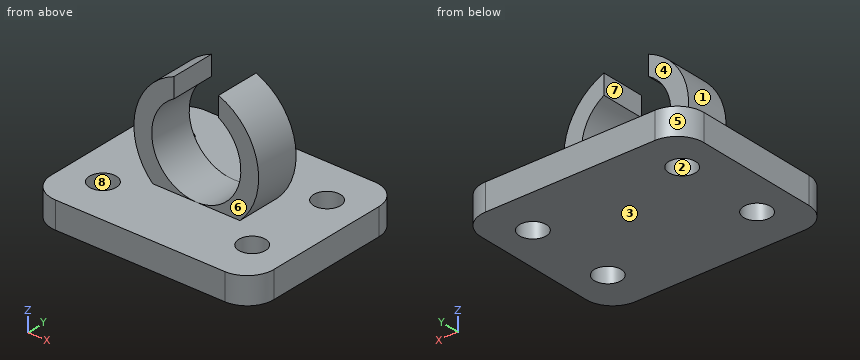
Autodesk Inventor part; units mm, degrees
ref_plane "YZ Plane" through (0, 0, 0) normal (1, 0, 0) x (0, 1, 0)
ref_plane "XZ Plane" through (0, 0, 0) normal (0, 1, 0) x (-1, 0, 0)
ref_plane "XY Plane" through (0, 0, 0) normal (0, 0, 1) x (1, 0, 0)
sketch "Szkic1" plane through (0, 0, 0) normal (0, 0, 1) x (1, 0, 0)
  line L0 (-12.5, -10) -> (12.5, -10)
  line L1 (12.5, -10) -> (12.5, 10)
  line L2 (12.5, 10) -> (-12.5, 10)
  line L3 (-12.5, 10) -> (-12.5, -10)
  line L4 (-12.5, -10) -> (12.5, 10) construction
  line L5 (12.5, -10) -> (-12.5, 10) construction
  point P0 (0, 0)
  dimension "d0" = 25
  dimension "d1" = 20
extrude "Wyciągnięcie proste1" add sketch "Szkic1" along normal blind 3
sketch "Szkic2" plane through (0, 0, 0) normal (0, 1, 0) x (-1, 0, 0)
  circle A0 centre (0, 8) radius 7
  line L0 (12.5, 3) -> (-12.5, 3)
  line L1 (12.5, 0) -> (-12.5, 0)
  circle A1 centre (0, 8) radius 5
  line L2 (4.899, 3) -> (-4.899, 3)
  point P0 (0, 0)
  point P1 (0, 0)
  dimension "d4" = 14
  dimension "d5" = 10
extrude "Wyciągnięcie proste2" add sketch "Szkic2" along normal mid plane 5 contours A0 L0 picked at (6.263, 8.5684)
sketch "Szkic3" plane through (-12.5, 10, 0) normal (0, 1, 0) x (1, 0, 0)
  line L0 (10, -16) -> (15, -16)
  line L1 (15, -16) -> (15, -12)
  line L2 (15, -12) -> (10, -12)
  line L3 (10, -12) -> (10, -16)
  line L4 (10, -16) -> (15, -12) construction
  line L5 (15, -16) -> (10, -12) construction
  circle A0 centre (12.5, -8) radius 5
  line L6 (25, 0) -> (0, 0)
  point P0 (12.5, 0)
  point P1 (12.5, -14)
  point P2 (12.5, -14)
  point P3 (12.5, 0)
  dimension "d8" = 5
  dimension "d9" = 4
  dimension "d10" = 6
extrude "Wyciągnięcie proste3" cut sketch "Szkic3" against normal blind 20 contours L3 A0 L1 L0 | L3 L2 L1 A0 picked at (12.3258, -12.3242)
sketch "Szkic5" plane through (0, 0, 0) normal (0, 0, -1) x (-1, 0, 0)
  line L0 (12.5, 10) -> (12.5, -10)
  line L1 (-12.5, 10) -> (12.5, 10)
  line L2 (-12.5, -10) -> (-12.5, 10)
  line L3 (-12.5, 0) -> (12.5, 0) construction
  line L4 (0, 10) -> (0, -10) construction
  line L5 (12.5, -10) -> (-12.5, -10)
  point P0 (0, 0)
  point P1 (8.375, 5)
  point P2 (8.375, -5)
  point P3 (-8.375, 5)
  point P4 (-8.375, -5)
  dimension "d22" = 4.125
  dimension "d23" = 5
hole "Otwór2" at (-8.375, 5, 0) at (-8.375, -5, 0) at (8.375, 5, 0) at (8.375, -5, 0) direction (0, 0, 1) diameter 3 end through all
fillet "Zaokrąglenie1" radius 3 4 edges at (-12.5, -10, 1.5) (-12.5, 10, 1.5) (12.5, 10, 1.5) (12.5, -10, 1.5)
properties part number "uchwyt_przewody"
Could you check a few things on this model? Use its own coordinates, in mm. Face numbers are marked on the shaded views. A direction names the side the tool comes from. Round coordinates to 2 decimals unless told otherwise and drop trailing zeros. Loops run counter-clockwise (first coordinate to the right, second up) from the corner with the lowest first, then second, coordinate; pieces in that order, holes last. Notation, with made-up numbers: (23, -7.75) - (53, -7.75) arc R34 ccw to (53, 26.25) - close; hole circle Ø11 at (-36, -12.5). An arc over 180 degrees is marked (long way). Answer in a Markdown table with one row per item. Add a question column.
(1) If we section it at B-B (z = 8): Please give me the cut outline in (x, y).
(2) If we mould it in two halves opening along Z, with no side actions, what happens to the marked faces 1, 2 and 3? For each: pulls with the +Z half, pulls with the -Z half, needs draft (parallel to the pull), parting line crosses it, or undercut.
(3) I need wall thicknesses on line 1 along X through (y, z) = (-5, 1.35) (3 decimals); line 2 along Y through (x, z) = (-9.75, 2); line 3 along Z through (x, y) = (0.75, 3). Which ranges of each line are inside material? Lowest first, please.
(4) If we section it at C-C (z = 2.25): Please give me the cut outline in (x, y) (3 decimals).
(5) I'm going to push flat-ended pins straight in: pin 1 (2.5 mm diameter, centred on x = 8.375, y = 5, fed in from -Z); pin 2 (8 mm diameter, centred on x = 9, y = 2, fed in from -Z); pin 3 (1 mm diameter, centred on y = 2.5, z = 12.5, fed in from +X); pin 4 (3.5 mm diameter, centred on x = 3, z = 11, fed in from +Y). Where does each tip first touch, or does it pass through?
(6) If we section it at A-A (y = 5): Please give me the cut outline in (x, z) (3 decimals), plus the area to 3 significant figures.
(7) For the marked faces 4, 5, 6, 7 and 8, which set-ups out of +Z, -Z, +X, -X, +Y, -Y let a thin tool reach every point of the face, with its end or its side?
Model answer:
| question | item | result |
|---|---|---|
| 1 | outline | (-7, -2.5) - (-5, -2.5) - (-5, 2.5) - (-7, 2.5) - close; (5, -2.5) - (7, -2.5) - (7, 2.5) - (5, 2.5) - close |
| 2 | face 1 | undercut |
| 2 | face 2 | needs draft |
| 2 | face 3 | pulls with the -Z half |
| 3 | line 1 | x = -12.5 to -9.875, -6.875 to 6.875, 9.875 to 12.5 |
| 3 | line 2 | y = -9.99 to -5.6, -4.4 to 4.4, 5.6 to 9.99 |
| 3 | line 3 | z = 0 to 3 |
| 4 | outline | (-12.5, -7) arc R3 ccw to (-9.5, -10) - (9.5, -10) arc R3 ccw to (12.5, -7) - (12.5, 7) arc R3 ccw to (9.5, 10) - (-9.5, 10) arc R3 ccw to (-12.5, 7) - close; hole circle Ø3 at (-8.375, -5); hole circle Ø3 at (-8.375, 5); hole circle Ø3 at (8.375, -5); hole circle Ø3 at (8.375, 5) |
| 5 | pin 1 | passes through |
| 5 | pin 2 | stops at z = 0 |
| 5 | pin 3 | stops at x = 5.74 |
| 5 | pin 4 | stops at y = 2.5 |
| 6 | outline | (-12.5, 0) - (-9.875, 0) - (-9.875, 3) - (-12.5, 3) - close; (-6.875, 0) - (6.875, 0) - (6.875, 3) - (-6.875, 3) - close; (9.875, 0) - (12.5, 0) - (12.5, 3) - (9.875, 3) - close |
| 6 | area | 57.0 mm² |
| 7 | face 4 | +Z, +X, -X, +Y |
| 7 | face 5 | +Z, -Z, -X, +Y |
| 7 | face 6 | +Z, +X, -X, -Y |
| 7 | face 7 | +Z, +Y, -Y |
| 7 | face 8 | +Z, -Z |
